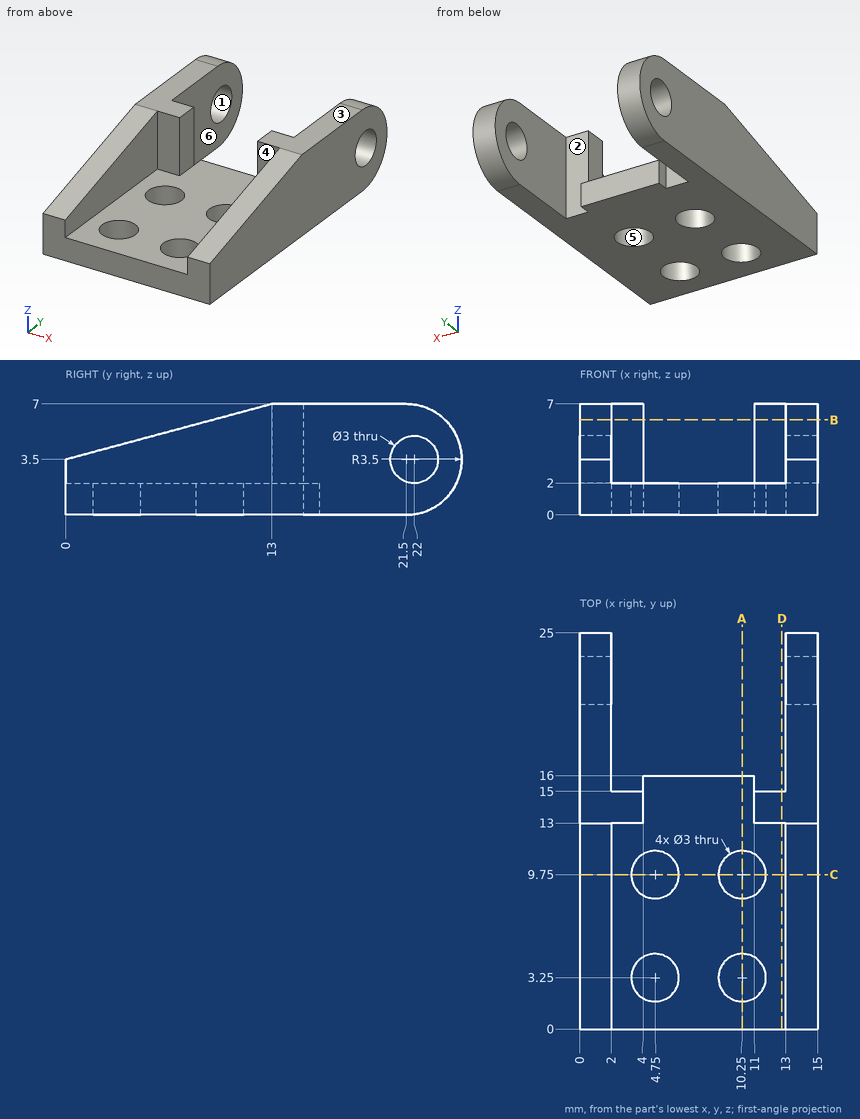
Here's the drawing with two shaded views (mm, measured from the low corner). I have some questions. A direction names the side the tool comes from. Round coordinates to 2 decimals unless told otherwise and drop trailing zeros. Loops run counter-clockwise (first coordinate to the right, second up) from the corner with the lowest first, then second, coordinate; pieces in that order, holes last.
1. Suppose I cut it at B-B, the plane z = 6. Please give me the cut outline in (x, y), and give its area (3 significant figures).
Answers:
outline: (0, 9.29) - (2, 9.29) - (2, 13) - (4, 13) - (4, 15) - (2, 15) - (2, 23.95) - (0, 23.95) - close; (11, 13) - (13, 13) - (13, 9.29) - (15, 9.29) - (15, 23.95) - (13, 23.95) - (13, 15) - (11, 15) - close
area: 66.7 mm2
2. Suppose I cut it at C-C, the plane y = 9.75. Please give me the cut outline in (x, z) (3 decimals), and give its area (3 significant figures).
Answers:
outline: (0, 0) - (3.25, 0) - (3.25, 2) - (2, 2) - (2, 6.125) - (0, 6.125) - close; (6.25, 0) - (8.75, 0) - (8.75, 2) - (6.25, 2) - close; (11.75, 0) - (15, 0) - (15, 6.125) - (13, 6.125) - (13, 2) - (11.75, 2) - close
area: 34.5 mm2
3. Will these pins go through, and if not, where does the flat tip stop? pin 1 (2.5 mm diameter, centred on y = 22, z = 3.5, fed in from -X); pin 2 (4 mm diameter, centred on x = 7.5, z = 1, fed in from +Y); pin 3 (5.5 mm diameter, centred on x = 9, y = 10, fed in from +Z); pin 4 (1 mm diameter, centred on x = 12, z = 4.5, fed in from +Y).
Answers:
pin 1: passes through
pin 2: stops at y = 16
pin 3: stops at z = 2
pin 4: stops at y = 15
4. If I drill on probe 1 along Y at (x, z) = (4.75, 1.1); probe 2 along X at (y, z) = (18.25, 0.5); probe 3 along Z at (x, y) = (2.5, 3.25), over which ranges is the centre line in solid material (lowest first)?
Answers:
probe 1: y = 0 to 1.75, 4.75 to 8.25, 11.25 to 16
probe 2: x = 0 to 2, 13 to 15
probe 3: z = 0 to 2
5. Suppose I cut it at A-A, the plane x = 10.25. Please give me the cut outline in (y, z).
Answers:
outline: (0, 0) - (1.75, 0) - (1.75, 2) - (0, 2) - close; (4.75, 0) - (8.25, 0) - (8.25, 2) - (4.75, 2) - close; (11.25, 0) - (16, 0) - (16, 2) - (11.25, 2) - close
6. Thinking about a two-plate mould opening in Y: for the marked faces 1, 2 and 3, which applies, released by +Y, released by -Y, zero draft, split by the parting line, or undercut?
Answers:
face 1: undercut
face 2: released by +Y
face 3: zero draft
7. For the marked faces 4, 5 and 6, which set-ups out of +Z, -Z, +X, -X, +Y, -Y let a thin tool reach every point of the face, with its end or its side?
Answers:
face 4: +Z, -Y
face 5: +Z, -Z
face 6: +Z, -Z, +Y
8. Suppose I cut it at D-D, the plane x = 12.75. Please give me the cut outline in (y, z), and give its area (3 significant figures).
Answers:
outline: (0, 0) - (15, 0) - (15, 7) - (13, 7) - (13, 2) - (0, 2) - close
area: 40.0 mm2
